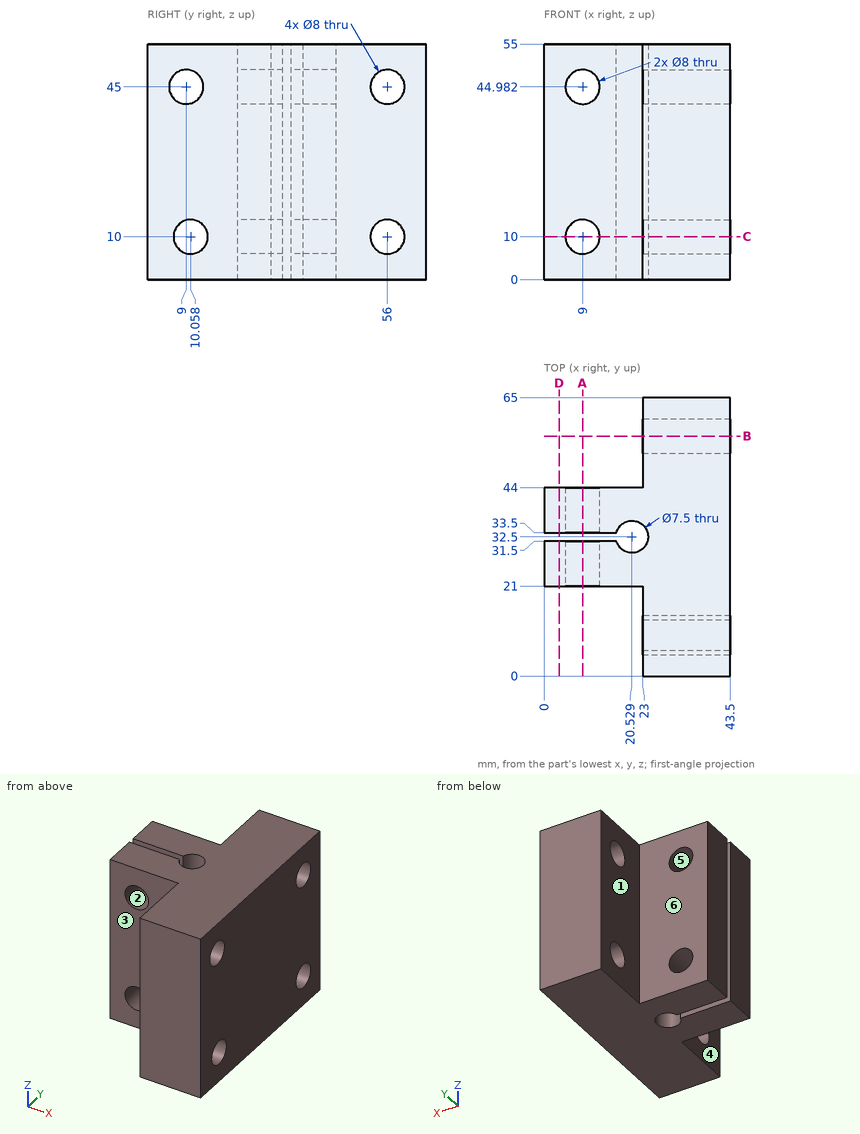
For this review, use the dimensioned drawing (mm, ordinates from the lowest corner) and the shaded views. A direction names the side the tool comes from. Round coordinates to 2 decimals unless told otherwise and drop trailing zeros. Write each loop counter-clockwise with the first axis right and the second up, starting at its lowest first coordinate (ties: lowest second). Pieces come first, ordered by that corner, then holes. Notation, with made-up numbers: (14, 31.5) - (68, 31.5) arc R3 cw to (68, 36.5) - close; hole circle Ø11 at (85, 68.25). An arc over 180 degrees is marked (long way). Answer as a JSON object with one key per item and string values.
1. Tool access review of the marked faces 1, 2 and 3: name each direction out of +Z, -Z, +X, -X, +Y, -Y from which nothing blocks a thin tool from reaching the whole face with its end or side.
Response values:
{"face 1": "+Z, -Z, -X, +Y", "face 2": "+Y, -Y", "face 3": "+Z, -Z, -X, -Y"}
2. We need section B-B on y = 56. Give the boundary of the cut face in (x, z).
Response values:
{"outline": "(23, 0) - (43.5, 0) - (43.5, 6) - (23, 6) - close; (23, 14) - (43.5, 14) - (43.5, 41) - (23, 41) - close; (23, 49) - (43.5, 49) - (43.5, 55) - (23, 55) - close"}
3. For pin 1 Ø5 at (x, y) = (25, 36) entering from -Z; pin 2 Ø13 at (x, z) = (9, 44.98) entering from +Y; pin 3 Ø17 at (y, z) = (54.5, 34.5) entering from -X; pin 4 Ø11.5 at (x, z) = (15.5, 41) entering from -Y, all flat-tipped, find the tip position at first contact; note any pin that passes through.
Response values:
{"pin 1": "stops at z = 0", "pin 2": "stops at y = 44", "pin 3": "stops at x = 23", "pin 4": "stops at y = 21"}
4. We need section C-C on z = 10. Count the separate pieces of the cut face and the enclosed holes in it, then the cut area to 3 significant figures.
Response values:
{"separate pieces": "5", "enclosed holes": "0", "area": "1,290 mm2"}
5. We need section A-A on x = 9. Give the boundary of the cut face in (y, z), then the cut area to 3 significant figures.
Response values:
{"outline": "(21, 0) - (31.5, 0) - (31.5, 6) - (21, 6) - close; (21, 14) - (31.5, 14) - (31.5, 40.98) - (21, 40.98) - close; (21, 48.98) - (31.5, 48.98) - (31.5, 55) - (21, 55) - close; (33.5, 0) - (44, 0) - (44, 6) - (33.5, 6) - close; (33.5, 14) - (44, 14) - (44, 40.98) - (33.5, 40.98) - close; (33.5, 48.98) - (44, 48.98) - (44, 55) - (33.5, 55) - close", "area": "819 mm2"}
6. To check wall thickness, follow line 1 along Z through (x, y) = (39.25, 56); line 2 along Z through (x, y) = (28.5, 54) (1 decimal); line 3 along Y through (x, z) = (16, 40.5). State the ranges of each line that lie inside material, in increasing order.
Response values:
{"line 1": "z = 0 to 6, 14 to 41, 49 to 55", "line 2": "z = 0 to 6.5, 13.5 to 41.5, 48.5 to 55", "line 3": "y = 21 to 31.5, 33.5 to 44"}
7. Draft analysis for pull direction X (two halves, no side actions). For the marked faces 4, 5 and 6, state which applies: +X half, -X half, draft (parallel to the pull), parting line (faces both ways), or undercut.
Response values:
{"face 4": "-X half", "face 5": "undercut", "face 6": "draft"}
8. We need section D-D on x = 3.5. Give the boundary of the cut face in (y, z).
Response values:
{"outline": "(21, 0) - (31.5, 0) - (31.5, 55) - (21, 55) - close; (33.5, 0) - (44, 0) - (44, 55) - (33.5, 55) - close"}
